```python
from build123d import *

# Parameters (mm, degrees)
F1_DEPTH  = 31.75
F3_DEPTH  = 50.801
F5_DEPTH  = 19.05
F7_DEPTH  = 19.05
F10_DEPTH = 25.4


with BuildPart() as f1:
    # F0 (on Front) → F1 (new body)
    with BuildSketch(Plane.XZ):
        Polygon((-15.0988876544, 54.272421198), (-65.8988876544, 53.8816550068), (-65.8988876544, 9.4316550068), (-15.0988876544, 9.4316550068), align=None)
    extrude(amount=F1_DEPTH)

    # F2 (on face) → F3 (cut, through all)
    with BuildSketch(Plane.YZ.offset(-15.0988876544)):
        Polygon((-12.7, 54.272421198), (-31.75, 54.272421198), (-31.75, 28.872421198), align=None)
    extrude(amount=-F3_DEPTH, mode=Mode.SUBTRACT)

    # F4 (on face) → F5 (cut)
    with BuildSketch(Plane.YZ.offset(-15.0988876544)):
        Polygon((-12.7, 54.272421198), (-31.75, 28.872421198), (-12.8411110491, 28.872421198), align=None)
    extrude(amount=-F5_DEPTH, mode=Mode.SUBTRACT)

    # F6 (on face) → F7 (cut)
    with BuildSketch(Plane(origin=(-65.8988876544, 0, 0), x_dir=(0, -1, 0), z_dir=(-1, 0, 0))):
        Polygon((31.75, 28.872421198), (12.9930746434, 53.8816550068), (12.9930746434, 28.872421198), align=None)
    extrude(amount=-F7_DEPTH, mode=Mode.SUBTRACT)

    # F8 (on face) + F9 (on face) → F10 (cut)
    with BuildSketch(Plane(origin=(0, -13.00111205, 0.0722283685), x_dir=(1, 0, 0), z_dir=(0, -0.9999845683, 0.0055554674))):
        Polygon((-15.0988876544, 28.800637273), (-15.0988876544, 54.201029245), (-27.7985119257, 54.1033390799), align=None)
    with BuildSketch(Plane(origin=(-0.4183455733, 0, 54.3853475663), x_dir=(0.999970416, 0, 0.0076920203), z_dir=(-0.0076920203, 0, 0.999970416))):
        Polygon((-27.4383474236, 0), (-27.4378046857, -12.700545143), (-14.6809764035, -12.7), (-14.6809764035, 0), align=None)
    extrude(amount=-F10_DEPTH, dir=(0, -0.9999845683, 0.0055554674), mode=Mode.SUBTRACT)


solid = f1.part
```
The model under review builds one solid part; all positions refer to its coordinate system, in mm. A direction names the side the tool comes from. Round coordinates to 2 decimals unless told otherwise and drop trailing zeros. Order: outer loops, then holes, each group sorted by start corner. A loop starts at its lowest first (then second) coordinate and runs counter-clockwise, first axis right, second up. Notation, with made-up numbers: M 12.25,82.5 L 41.25,82.5 A23 ccw 41.25,119.5 Z; hole C 54.25,45.25 d10. An arc over 180 degrees is marked long. Use a Markdown table: item, result.
1) Draft analysis for pull direction Y (two halves, no side actions). For faces 4 (the face through (-34.149, -18, 36)), 5 (the face through (-41, 0, 32)), 6 (the face through (-41, -31.75, 19)), state which applies: released by +Y, released by -Y, zero draft, split by the parting line, or undercut.
Report:
| item | result |
|---|---|
| face 4 | zero draft |
| face 5 | released by +Y |
| face 6 | released by -Y |
2) Consider section D-D (y = -28). Write out the cut boundary in (x, z).
Report:
| item | result |
|---|---|
| outline | M -65.9,9.43 L -15.1,9.43 L -15.1,28.87 L -34.15,28.87 L -34.15,33.87 L -46.85,33.87 L -46.85,28.87 L -65.9,28.87 Z |
3) Insertion check: pin 1 (5 mm diameter, centred on x = -37.5, y = -11.5, fed in from +Z); pin 2 (8 mm diameter, centred on x = -26.5, z = 33, fed in from -Y); pin 3 (15 mm diameter, centred on x = -26.5, y = -27, fed in from +Z). Each pin has a flat end and moves straight along its axis. Give the tip position at first contact, or say it passes through.
Report:
| item | result |
|---|---|
| pin 1 | z = 54.12 |
| pin 2 | y = -12.84 |
| pin 3 | z = 28.87 |
4) Consider section C-C (x = -60.5). Write out the cut boundary in (y, z), then the cut area to 3 significant figures.
Report:
| item | result |
|---|---|
| outline | M -31.75,9.43 L 0,9.43 L 0,53.92 L -12.96,53.92 L -12.99,53.88 L -12.99,28.87 L -31.75,28.87 Z |
| area | 943 mm^2 |
5) Tool access review of faces 1 (the face through (-41, -16, 9.432)), 2 (the face through (-24, -22, 28.872)), 3 (the face through (-57, -22, 28.872)): name each direction out of +Z, -Z, +X, -X, +Y, -Y from which nothing blocks a thin tool from reaching the whole face with its end or side.
Report:
| item | result |
|---|---|
| face 1 | -Z, +X, -X, +Y, -Y |
| face 2 | +Z, +X, -Y |
| face 3 | +Z, -X, -Y |
6) Consider section B-B (z = 48.5). Write out the cut boundary in (x, y), then the cut area to 3 significant figures.
Report:
| item | result |
|---|---|
| outline | M -65.9,-12.99 L -46.85,-12.99 L -46.85,-17.03 L -34.15,-17.03 L -34.15,-12.73 L -24.95,-12.73 L -24.99,0 L -65.9,0 Z |
| area | 581 mm^2 |
7) Wall thickness on line 1 along X through (y, z) = (-14.5, 34); line 2 along Z through (x, y) = (-39, -11); line 3 along Y through (x, z) = (-33.5, 32): over which ranges is each line inside the solid? List them lowest first. Write a range as [from, to].
Report:
| item | result |
|---|---|
| line 1 | [-46.85, -34.15] |
| line 2 | [9.43, 54.09] |
| line 3 | [-12.82, 0] |
